from build123d import *

# Parameters (mm, degrees)
F0_W     = 34.8
F0_H     = 28
F1_DEPTH = 2.5
F2_W     = 32.8
F2_H     = 26
F3_DEPTH = 1.5
F4_W     = 6
F4_H     = 28
F5_DEPTH = 1.5


with BuildPart() as f1:
    # F0 (on Top) → F1 (new body)
    with BuildSketch(Plane.XY):
        Rectangle(F0_W, F0_H)
    extrude(amount=F1_DEPTH)

    # F2 (on face) → F3 (cut)
    with BuildSketch(Plane.XY.offset(2.5)):
        Rectangle(F2_W, F2_H)
    extrude(amount=-F3_DEPTH, mode=Mode.SUBTRACT)

    # F4 (on face) → F5 (cut)
    with BuildSketch(Plane.XY.offset(1)):
        with Locations((-8.4, 0)):
            Rectangle(F4_W, F4_H)
    extrude(amount=F5_DEPTH, mode=Mode.SUBTRACT)


solid = f1.part
Geometry: final body of the model. Coordinates: model frame, mm. A direction names the side the tool comes from. Coordinates: 2 decimals unless noted, no trailing zeros. Loops run counter-clockwise (first coordinate to the right, second up) from the corner with the lowest first, then second, coordinate; pieces in that order, holes last. Notation, with made-up numbers: (5, 25) - (62, 25) arc R19 ccw to (62, 58) - close; hole circle Ø3 at (41.5, -31). An arc over 180 degrees is marked (long way). Put each result on its own line as item: value. Start each with the question number.
Q1. Cut plane C-C, the plane x = -2.5. Return loops of the section in (y, z).
Q2. Pin query (flat end, axial travel): pin 1 Ø8 at (x, y) = (-6, -9) entering from -Z; pin 2 Ø6 at (x, y) = (0, -1) entering from +Z. Return the tip coordinate at first contact, or that it passes through.
Q3. Cut plane D-D, the plane x = -8. Return loops of the section in (y, z), and give its area (3 significant figures).
Q4. Set-up query: faces 1 (the flat face through (-16.4, 0, 2)), 2 (the flat face through (0, 0, 0)), 3 (the flat face through (-11.4, -13.5, 1.7)). Return all of +Z, -Z, +X, -X, +Y, -Y with unobstructed straight access to the full face (end or side cutting, diameter ignored); none if empty.
Q5. Cut plane B-B, the plane y = 11.5. Return loops of the section in (x, z), and give its area (3 significant figures).
Q6. Cut plane A-A, the plane z = 1.6. Return loops of the section in (x, y).
Q7. Pull-direction query (X, two-part tool) for faces 4 (the flat face through (17, 0, 2.5)), 5 (the flat face through (5, 13, 2)), 6 (the flat face through (-17.4, 0, 1)), 7 (the flat face through (-5.4, 13.5, 1.7)); classes: released by +X, released by -X, zero draft, split by the parting line, or undercut.
Q8. Line query: line 1 (X direction, y = -1.5, z = 1.7); line 2 (Y direction, x = 2.5, z = 1.55); line 3 (Z direction, x = -11.5, y = 8.25). Output: solid intervals per line, ascending.
Filled sheet:
1. outline: (-14, 0) - (14, 0) - (14, 2.5) - (13, 2.5) - (13, 1) - (-13, 1) - (-13, 2.5) - (-14, 2.5) - close
2. pin 1: z = 0
2. pin 2: z = 1
3. outline: (-14, 0) - (14, 0) - (14, 1) - (-14, 1) - close
3. area: 28.0 mm²
4. face 1: +Z
4. face 2: -Z, +X, -X, +Y, -Y
4. face 3: +Z, +Y, -Y
5. outline: (-17.4, 0) - (17.4, 0) - (17.4, 2.5) - (16.4, 2.5) - (16.4, 1) - (-16.4, 1) - (-16.4, 2.5) - (-17.4, 2.5) - close
5. area: 37.8 mm²
6. outline: (-17.4, -14) - (-11.4, -14) - (-11.4, -13) - (-16.4, -13) - (-16.4, 13) - (-11.4, 13) - (-11.4, 14) - (-17.4, 14) - close; (-5.4, -14) - (17.4, -14) - (17.4, 14) - (-5.4, 14) - (-5.4, 13) - (16.4, 13) - (16.4, -13) - (-5.4, -13) - close
7. face 4: zero draft
7. face 5: undercut
7. face 6: released by -X
7. face 7: undercut
8. line 1: -17.4 to -16.4, 16.4 to 17.4
8. line 2: -14 to -13, 13 to 14
8. line 3: 0 to 1
